Source: CAD feature listing. Evaluate the final solid. Frame: model axes, mm. A direction names the side the tool comes from. Coordinates: 2 decimals unless noted, no trailing zeros. Loops run counter-clockwise (first coordinate to the right, second up) from the corner with the lowest first, then second, coordinate; pieces in that order, holes last. Notation, with made-up numbers: (41, 50) - (85, 50) arc R24 ccw to (85, 83) - close; hole circle Ø1 at (22, -13.5). An arc over 180 degrees is marked (long way). Write item = value, one per line. Start each with the question number.
from build123d import *

# Parameters (mm, degrees)
ESBO_O1_W                                    = 203
ESBO_O1_H                                    = 116
RESSALTO_EXTRUS_O1_DEPTH                     = 6
ESBO_O2_W                                    = 194
ESBO_O2_H                                    = 112
CORTE_EXTRUS_O1_DEPTH                        = 1
FILETE2_R                                    = 3
ESBO_O3_W                                    = 174
ESBO_O3_H                                    = 109
RESSALTO_EXTRUS_O2_DEPTH                     = 11
ESBO_O4_W                                    = 110
ESBO_O4_H                                    = 109
CORTE_EXTRUS_O2_DEPTH                        = 6
ESBO_O5_W                                    = 170
ESBO_O5_H                                    = 105
CORTE_EXTRUS_O3_DEPTH                        = 8
FURO_COM_FOLGA_DE_M31_D                      = 3.4
ESCAREADO_PARA_PARAFUSO_COM_CABE_A_E_2_COUNT = 2
ESCAREADO_PARA_PARAFUSO_COM_CABE_A_E_2_PITCH = 155
ESCAREADO_PARA_PARAFUSO_COM_CABE_A_E_3_COUNT = 2
ESCAREADO_PARA_PARAFUSO_COM_CABE_A_E_3_PITCH = 70
ESCAREADO_PARA_PARAFUSO_COM_CABE_A_E_4_COUNT = 2
ESCAREADO_PARA_PARAFUSO_COM_CABE_A_E_4_PITCH = 170.073513517
ESBO_O10_W                                   = 30
ESBO_O10_H                                   = 10
RESSALTO_EXTRUS_O3_DEPTH                     = 3
FILETE3_R                                    = 10


with BuildPart() as part:
    # Esboço1 → Ressalto-extrusão1 (new body)
    with BuildSketch(Plane.XY):
        Rectangle(ESBO_O1_W, ESBO_O1_H)
    extrude(amount=RESSALTO_EXTRUS_O1_DEPTH)

    # Esboço2 → Corte-extrusão1 (cut)
    with BuildSketch(Plane.XY.offset(6)):
        Rectangle(ESBO_O2_W, ESBO_O2_H)
    extrude(amount=-CORTE_EXTRUS_O1_DEPTH, mode=Mode.SUBTRACT)

    # Filete2
    filete2_edges = [part.edges().sort_by_distance(p)[0] for p in [
        (-101.5, 0, 6),
        (101.5, 0, 6),
    ]]
    fillet(filete2_edges, radius=FILETE2_R)

    # Esboço3 → Ressalto-extrusão2 (add)
    with BuildSketch(Plane(origin=(0, 0, 5), x_dir=(-1, 0, 0), z_dir=(0, 0, -1))):
        Rectangle(ESBO_O3_W, ESBO_O3_H)
    extrude(amount=RESSALTO_EXTRUS_O2_DEPTH)

    # Esboço4 → Corte-extrusão2 (cut)
    with BuildSketch(Plane(origin=(0, 0, -6), x_dir=(-1, 0, 0), z_dir=(0, 0, -1))):
        Rectangle(ESBO_O4_W, ESBO_O4_H)
    extrude(amount=-CORTE_EXTRUS_O2_DEPTH, mode=Mode.SUBTRACT)

    # Esboço5 → Corte-extrusão3 (cut)
    with BuildSketch(Plane.XY.offset(5)):
        Rectangle(ESBO_O5_W, ESBO_O5_H)
    extrude(amount=-CORTE_EXTRUS_O3_DEPTH, mode=Mode.SUBTRACT)

    # Furo com folga de M31 (through all)
    with Locations(Plane(origin=(0, 0, -6), x_dir=(-1, 0, 0), z_dir=(0, 0, -1))):
        with Locations((-63, 33), (63, 33), (63, -33), (-63, -33)):
            Hole(FURO_COM_FOLGA_DE_M31_D / 2)

    # Esboço9 → Escareado para parafuso com cabeça escareada chata de M41 (revolve, cut)
    with BuildSketch(Plane(origin=(77.5, 35, -3), x_dir=(0, -1, 0), z_dir=(1, 0, 0))):
        Polygon((0, 0), (0, 3), (2.25, 3), (2.25, 2.45), (4.7, 0), align=None)
    escareado_para_parafuso_com_cabe_a_escar = revolve(axis=Axis((77.5, 35, 3.35), (0, 0, -1)), mode=Mode.SUBTRACT)

    # Escareado para parafuso com cabe_a e 2: Escareado para parafuso com cabeça escareada chata de M41 ×2
    with Locations(*[(-i * ESCAREADO_PARA_PARAFUSO_COM_CABE_A_E_2_PITCH, 0, 0) for i in range(1, ESCAREADO_PARA_PARAFUSO_COM_CABE_A_E_2_COUNT)]):
        add(escareado_para_parafuso_com_cabe_a_escar, mode=Mode.SUBTRACT)

    # Escareado para parafuso com cabe_a e 3: Escareado para parafuso com cabeça escareada chata de M41 ×2
    with Locations(*[(0, -i * ESCAREADO_PARA_PARAFUSO_COM_CABE_A_E_3_PITCH, 0) for i in range(1, ESCAREADO_PARA_PARAFUSO_COM_CABE_A_E_3_COUNT)]):
        add(escareado_para_parafuso_com_cabe_a_escar, mode=Mode.SUBTRACT)

    # Escareado para parafuso com cabe_a e 4: Escareado para parafuso com cabeça escareada chata de M41 ×2
    with Locations(*[Vector(-0.911370599658675, -0.41158672242649835, 0) * (i * ESCAREADO_PARA_PARAFUSO_COM_CABE_A_E_4_PITCH) for i in range(1, ESCAREADO_PARA_PARAFUSO_COM_CABE_A_E_4_COUNT)]):
        add(escareado_para_parafuso_com_cabe_a_escar, mode=Mode.SUBTRACT)

    # Esboço10 → Ressalto-extrusão3 (add)
    with BuildSketch(Plane.XY.offset(-3)):
        with Locations((-70, 47.5)):
            Rectangle(ESBO_O10_W, ESBO_O10_H)
        with Locations((70, 47.5)):
            Rectangle(ESBO_O10_W, ESBO_O10_H)
        with Locations((70, -47.5)):
            Rectangle(ESBO_O10_W, ESBO_O10_H)
        with Locations((-70, -47.5)):
            Rectangle(ESBO_O10_W, ESBO_O10_H)
    extrude(amount=RESSALTO_EXTRUS_O3_DEPTH)

    # Filete3
    filete3_edges = [part.edges().sort_by_distance(p)[0] for p in [
        (-85, 42.5, -1.5),
        (85, 42.5, -1.5),
        (85, -42.5, -1.5),
        (-85, -42.5, -1.5),
    ]]
    fillet(filete3_edges, radius=FILETE3_R)


solid = part.part
Item 1: First-contact query: pin 1 (3 mm diameter, centred on y = 39.5, z = -3.5, fed in from +X); pin 2 (2 mm diameter, centred on x = 63, y = 33, fed in from +Z); pin 3 (3 mm diameter, centred on x = -67.5, z = -2, fed in from +Y); pin 4 (5 mm diameter, centred on x = -77.5, y = 35, fed in from +Z). Flat tips, straight axial feed; report the tip coordinate or a pass-through.
Item 2: Reachability of faces 5 (the flat face through (70, -47, 0)), 6 (the cylindrical face through (-75.304, 35.488, -5.721)), 7 (the flat face through (71, 54.5, -3)) from +Z, -Z, +X, -X, +Y, -Y: full face, straight path, thin tool, end or side. Return the list, or none.
Item 3: Cut plane D-D (y = 10). Return the cut outline in (x, z), then the cut area to 3 significant figures.
Item 4: Cut plane B-B (y = 47.5). Return the cut outline in (x, z).
Item 5: Cut plane C-C (x = 58.5). Return the cut outline in (y, z), then the cut area to 3 significant figures.
Item 6: Draft query along X for faces 1 (the flat face through (-1, -52.5, 3)), 2 (the flat face through (-71, 1, -6)), 3 (the flat face through (-87, -1, -3)), 4 (the flat face through (87, -1, -3)). Return one class per face: released by +X, released by -X, zero draft, split by the parting line, or undercut.
Item 7: Material intervals for L1, parallel to Y at x = -77.5, z = -5.85; L2, parallel to X at y = -35, z = -5.8; L3, parallel to X at y = -48, z = -2.5, sorted ascending. Write a range as [from, to].
Item 8: Cut plane A-A (x = -13). Return the cut outline in (y, z).
Responses:
q1.pin_1 = 87
q1.pin_2 = through
q1.pin_3 = 54.5
q1.pin_4 = -5.2
q2.face_5 = +Z
q2.face_6 = +Z, -Z
q2.face_7 = -Z, +X, -X, +Y
q3.outline = (-101.5, 0) - (-87, 0) - (-87, -6) - (-55, -6) - (-55, -3) - (-85, -3) - (-85, 5) - (-97, 5) - (-97, 6) - (-98.5, 6) arc R3 ccw to (-101.5, 3) - close; (55, -6) - (87, -6) - (87, 0) - (101.5, 0) - (101.5, 3) arc R3 ccw to (98.5, 6) - (97, 6) - (97, 5) - (85, 5) - (85, -3) - (55, -3) - close
q3.area = 374 mm2
q4.outline = (-101.5, 0) - (-87, 0) - (-87, -6) - (-55, -6) - (-55, 0) - (-85, 0) - (-85, 5) - (-97, 5) - (-97, 6) - (-98.5, 6) arc R3 ccw to (-101.5, 3) - close; (55, -6) - (87, -6) - (87, 0) - (101.5, 0) - (101.5, 3) arc R3 ccw to (98.5, 6) - (97, 6) - (97, 5) - (85, 5) - (85, 0) - (55, 0) - close
q5.outline = (-58, 0) - (-54.5, 0) - (-54.5, -6) - (54.5, -6) - (54.5, 0) - (58, 0) - (58, 6) - (56, 6) - (56, 5) - (52.5, 5) - (52.5, 0) - (42.5, 0) - (42.5, -3) - (-42.5, -3) - (-42.5, 0) - (-52.5, 0) - (-52.5, 5) - (-56, 5) - (-56, 6) - (-58, 6) - close
q5.area = 458 mm2
q6.face_1 = undercut
q6.face_2 = zero draft
q6.face_3 = released by -X
q6.face_4 = released by +X
q7.L1 = [-54.5, -37.25], [-32.75, 32.75], [37.25, 54.5]
q7.L2 = [-87, -79.75], [-75.25, -55], [55, 75.25], [79.75, 87]
q7.L3 = [-87, -55], [55, 87]
q8.outline = (-58, 0) - (-52.5, 0) - (-52.5, 5) - (-56, 5) - (-56, 6) - (-58, 6) - close; (52.5, 0) - (58, 0) - (58, 6) - (56, 6) - (56, 5) - (52.5, 5) - close
